Verification items for the finished model (mm, model axes). Face numbers are marked on the shaded views. A direction names the side the tool comes from. Round coordinates to 2 decimals unless told otherwise and drop trailing zeros. Order: outer loops, then holes, each group sorted by start corner. A loop starts at its lowest first (then second) coordinate and runs counter-clockwise, first axis right, second up. Notation, with made-up numbers: M -25.75,-36 L -14.75,-36 A13 cw -14.75,-26 Z; hole C 17,31 d9. An arc over 180 degrees is marked long. Return JSON: item names as keys, results as strings. Group by question number.
from build123d import *

# Parameters (mm, degrees)
SKETCH1_R           = 40.34
BOSS_EXTRUDE1_DEPTH = 8
SKETCH2_R           = 7.5
BOSS_EXTRUDE2_DEPTH = 20
BOSS_EXTRUDE3_DEPTH = 10
SKETCH4_R           = 6
BOSS_EXTRUDE4_DEPTH = 50


with BuildPart() as part:
    # Sketch1 → Boss-Extrude1 (new body)
    with BuildSketch(Plane(origin=(0, 0, 0), x_dir=(1, 0, 0), z_dir=(0, 1, 0))):
        with Locations(Location((0, 0, 0), (0, 0, 270))):
            Circle(SKETCH1_R)
    extrude(amount=-BOSS_EXTRUDE1_DEPTH)

    # Sketch2 → Boss-Extrude2 (add)
    with BuildSketch(Plane(origin=(0, 0, 0), x_dir=(1, 0, 0), z_dir=(0, 1, 0))):
        with Locations(Location((0, 0, 0), (0, 0, 270))):
            Circle(SKETCH2_R)
    extrude(amount=BOSS_EXTRUDE2_DEPTH)

    # Sketch3 → Boss-Extrude3 (add)
    with BuildSketch(Plane.XZ.offset(8)):
        with BuildLine():
            ThreePointArc((11.103712575, 16.634529361), (-20, 0), (11.103712575, -16.634529361))
            ThreePointArc((11.103712575, -16.634529361), (4.84, 0), (11.103712575, 16.634529361))
        make_face()
    extrude(amount=BOSS_EXTRUDE3_DEPTH)

    # Sketch4 → Boss-Extrude4 (add)
    with BuildSketch(Plane.XZ.offset(8)):
        with Locations(Location((30.06, 0, 0), (0, 0, 90))):
            Circle(SKETCH4_R)
    extrude(amount=BOSS_EXTRUDE4_DEPTH)


solid = part.part
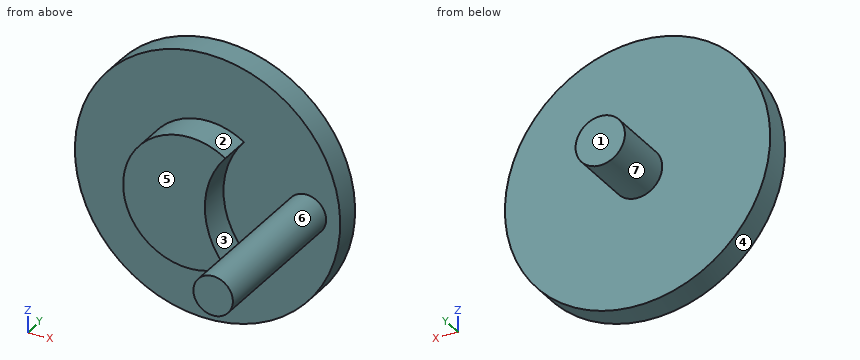
1. Cross-section at B-B (y = -13). Enter the section's corners in (x, z).
2. Access from +Z, -Z, +X, -X, +Y, -Y to the whole of each face (thin tool, end or side, straight path). Record for the marked faces 4, 5, 6 and 7.
3. Go/stop test with flat-tipped pins: pin 1 (10 mm diameter, centred on x = -30, z = -6.5, fed in from +Y); pin 2 (15.5 mm diameter, centred on x = -4.5, z = 0, fed in from -Y); pin 3 (4 mm diameter, centred on x = -31, z = 15, fed in from -Y). Record where each tip stops, or that it passes through.
4. Thickness scan on line 1 along Y through (x, z) = (10.5, 22.5); line 2 along Y through (x, z) = (-1.5, -5.5); line 3 along X through (y, z) = (10.5, -0.5). Record the ranges inside material, lowest first. Write a range as from..to.
5. Cross-section at D-D (y = 15.5). Enter the section's corners in (x, z), plus the area to 3 significant figures.
6. Draft check along X on the marked faces 1, 2 and 3. Enter one of: +X half, -X half, draft (parallel to the pull), parting line (faces both ways), or undercut.
7. Cross-section at C-C (z = -15). Enter the section's corners in (x, y), plus the area to 3 significant figures.
8. Cross-section at A-A (x = 0). Enter the section's corners in (y, z), plus the area to 3 significant figures.
Computed:
{
 "1": {"outline": "M 11.1,-16.63 A25.22 cw 11.1,16.63 A20 ccw long Z; C 30.06,0 d12"},
 "2": {"face 4": "+Y, -Y", "face 5": "+Z, -Z, -X, -Y", "face 6": "-Y", "face 7": "+Y"},
 "3": {"pin 1": "stops at y = 0", "pin 2": "stops at y = -18", "pin 3": "stops at y = -8"},
 "4": {"line 1": "y = -8..0", "line 2": "y = -18..20", "line 3": "x = -7.48..7.48"},
 "5": {"outline": "C 0,0 d15", "area": "177 mm²"},
 "6": {"face 1": "draft", "face 2": "parting line", "face 3": "undercut"},
 "7": {"outline": "M -37.45,-8 L -13.23,-8 L -13.23,-18 L 9.79,-18 L 9.79,-8 L 37.45,-8 L 37.45,0 L -37.45,0 Z", "area": "829 mm²"},
 "8": {"outline": "M -18,-20 L -8,-20 L -8,-40.34 L 0,-40.34 L 0,-7.5 L 20,-7.5 L 20,7.5 L 0,7.5 L 0,40.34 L -8,40.34 L -8,20 L -18,20 Z", "area": "1,350 mm²"}
}
